Geometry check sheet. Reference: the model listing, model coordinates, mm. A direction names the side the tool comes from. Round coordinates to 2 decimals unless told otherwise and drop trailing zeros. Order: outer loops, then holes, each group sorted by start corner. A loop starts at its lowest first (then second) coordinate and runs counter-clockwise, first axis right, second up. Notation, with made-up numbers: (6, 87.5) - (50, 87.5) arc R16 ccw to (50, 99.5) - close; hole circle Ø2 at (55, 17.25). An arc over 180 degrees is marked (long way). Use a Markdown table: item, result. Add a question column.
(1) Section check C-C on y = 2.7. Record the boundary of the cut face in (x, z).
(2) Section check D-D on x = 60. Record the boundary of the cut face in (y, z), then the cut area to 3 significant figures.
(3) Section check A-A on x = 68. Record the boundary of the cut face in (y, z).
(4) Access from +Z, -Z, +X, -X, +Y, -Y to the whole of each face (thin tool, end or side, straight path). Record for faces 1 (the face through (65.2, 1.6, -0.1)), 2 (the face through (-2.539, 3.479, 1.947)).
(5) Mould release check, pull along Z, two halves, no side actions. Record for faces 3 (the face through (-1.27, 3.07, 0.97)), 4 (the face through (32, 2, 0)), 5 (the face through (-7.5, 1.59, -0.16)): released by +Z, released by -Z, zero draft, split by the parting line, or undercut.
(6) Gauge pin test, flat ends, axial feed: P1, Ø3, axis at x = 46, z = 3.5, coming from the +Y side; P2, Ø2, axis at x = 52, y = 4, coming from the -Z side; P3, Ø2, axis at x = 3.5, y = 4.5, coming from the -Z side; P4, Ø3.5, axis at x = 0, z = 0, coming from the -Y side. Record the tip position at first contact, or that the pin passes through.
(7) Section check B-B on z = 0. Record the boundary of the cut face in (x, y).
(8) Thickness scan on line 1 along X through (y, z) = (1.75, 0); line 2 along Z through (x, y) = (68, 1.8); line 3 along X through (y, z) = (3.8, 0). Record the ranges inside material, lowest first. Write a range as [from, to].
```python
from build123d import *

# Parameters (mm, degrees)
BOSS_EXTRUDE1_DEPTH = 2
SKETCH2_R           = 1.6
CUT_EXTRUDE1_DEPTH  = 1.8
SKETCH3_R           = 0.8
CUT_EXTRUDE2_DEPTH  = 3
SKETCH4_R           = 2.8
CUT_EXTRUDE3_DEPTH  = 1.4
SKETCH5_R           = 3.2
SKETCH5_R_2         = 1.6
BOSS_EXTRUDE2_DEPTH = 3
SKETCH6_W           = 80.029728654
SKETCH6_H           = 15
CUT_EXTRUDE4_DEPTH  = 1.2


with BuildPart() as part:
    # Sketch1 → Boss-Extrude1 (new body)
    with BuildSketch(Plane(origin=(0, 0, 0), x_dir=(1, 0, 0), z_dir=(0, 1, 0))):
        with BuildLine():
            ThreePointArc((7.5, 0), (5.303300859, -5.303300859), (0, -7.5))
            Line((0, -7.5), (72, -7.5))
            Line((72, -7.5), (72, 7.5))
            Line((72, 7.5), (0, 7.5))
            ThreePointArc((0, 7.5), (5.303300859, 5.303300859), (7.5, 0))
        make_face()
        with BuildLine():
            ThreePointArc((0, 7.5), (-7.5, 0), (0, -7.5))
            Line((0, -7.5), (0, 7.5))
        make_face()
        with BuildLine():
            Line((0, 7.5), (0, -7.5))
            ThreePointArc((0, -7.5), (5.303300859, -5.303300859), (7.5, 0))
            ThreePointArc((7.5, 0), (5.303300859, 5.303300859), (0, 7.5))
        make_face()
    extrude(amount=BOSS_EXTRUDE1_DEPTH)

    # Sketch2 → Cut-Extrude1 (cut)
    with BuildSketch(Plane(origin=(0, 2, 0), x_dir=(1, 0, 0), z_dir=(0, 1, 0))):
        Circle(SKETCH2_R)
    extrude(amount=-CUT_EXTRUDE1_DEPTH, mode=Mode.SUBTRACT)

    # Sketch3 → Cut-Extrude2 (cut)
    with BuildSketch(Plane(origin=(0, 0.2, 0), x_dir=(1, 0, 0), z_dir=(0, 1, 0))):
        Circle(SKETCH3_R)
    extrude(amount=-CUT_EXTRUDE2_DEPTH, mode=Mode.SUBTRACT)

    # Sketch4 → Cut-Extrude3 (cut)
    with BuildSketch(Plane(origin=(0, 2, 0), x_dir=(1, 0, 0), z_dir=(0, 1, 0))):
        with Locations((68, 0)):
            Circle(SKETCH4_R)
    extrude(amount=-CUT_EXTRUDE3_DEPTH, mode=Mode.SUBTRACT)

    # Sketch5 → Boss-Extrude2 (add)
    with BuildSketch(Plane(origin=(0, 2, 0), x_dir=(1, 0, 0), z_dir=(0, 1, 0))):
        Circle(SKETCH5_R)
        Circle(SKETCH5_R_2, mode=Mode.SUBTRACT)
    extrude(amount=BOSS_EXTRUDE2_DEPTH)

    # Sketch6 → Cut-Extrude4 (cut)
    with BuildSketch(Plane.XZ):
        with Locations((31.985135673, 0)):
            Rectangle(SKETCH6_W, SKETCH6_H)
    extrude(amount=-CUT_EXTRUDE4_DEPTH, mode=Mode.SUBTRACT)


solid = part.part
```
Check sheet entries:
| question | item | result |
|---|---|---|
| 1 | outline | circle Ø6.4 at (0, 0); hole circle Ø3.2 at (0, 0) |
| 2 | outline | (1.2, -7.5) - (2, -7.5) - (2, 7.5) - (1.2, 7.5) - close |
| 2 | area | 12.0 mm2 |
| 3 | outline | (1.2, -7.5) - (2, -7.5) - (2, -2.8) - (1.2, -2.8) - close; (1.2, 2.8) - (2, 2.8) - (2, 7.5) - (1.2, 7.5) - close |
| 4 | face 1 | +Y, -Y |
| 4 | face 2 | +Y |
| 5 | face 3 | undercut |
| 5 | face 4 | zero draft |
| 5 | face 5 | split by the parting line |
| 6 | P1 | stops at y = 2 |
| 6 | P2 | passes through |
| 6 | P3 | stops at z = -2 |
| 6 | P4 | stops at y = 1.2 |
| 7 | outline | (-7.5, 1.2) - (-1.6, 1.2) - (-1.6, 5) - (-3.2, 5) - (-3.2, 2) - (-7.5, 2) - close; (1.6, 1.2) - (65.2, 1.2) - (65.2, 2) - (3.2, 2) - (3.2, 5) - (1.6, 5) - close; (70.8, 1.2) - (72, 1.2) - (72, 2) - (70.8, 2) - close |
| 8 | line 1 | x = [-7.5, -1.6], [1.6, 65.2], [70.8, 72] |
| 8 | line 2 | z = [-7.5, -2.8], [2.8, 7.5] |
| 8 | line 3 | x = [-3.2, -1.6], [1.6, 3.2] |
